Answer from the drawing. Dimensions are ordinates in mm from the lowest x, y and z of the part. Give positions to 0.01 mm unless a question says otherwise; leave off trailing zeros. Loops run counter-clockwise (first coordinate to the right, second up) from the corner with the lowest first, then second, coordinate; pieces in that order, holes last.
Item 1: The mould has two halves that part along Y. Classify the marked faces 1 and 2: pulls with the +Y half, pulls with the -Y half, needs draft (parallel to the pull), parting line crosses it, or undercut.
Item 2: Section A-A, the plane y = 15 is taken. Give the vertices of the cut face in (x, z), and give its area (3 significant figures).
Item 3: Section C-C, the plane z = 2.85 is taken. Give the vertices of the cut face in (x, y), and give its area (3 significant figures).
Item 4: Section D-D, the plane y = 69 is taken. Give the vertices of the cut face in (x, z), and give its area (3 significant figures).
Item 5: Section B-B, the plane x = 15 is taken. Give the vertices of the cut face in (y, z), and give its area (3 significant figures).
Item 6: Consider line 1 along Y through (x, z) = (15, 2.7); line 2 along Y through (x, z) = (10, 4.65); line 3 along X through (y, z) = (72.5, 3.7). Determine where each line is inside the solid, lowest interval first.
Item 7: Each of these flat-tipped pins is pushed along its axis until it touches: pin 1 Ø12 at (x, y) = (15, 15) entering from +Z; pin 2 Ø1 at (y, z) = (52, 3) entering from -X; pin 3 Ø3 at (y, z) = (68, 3) entering from +X. Where does it stop, or does it pass through?
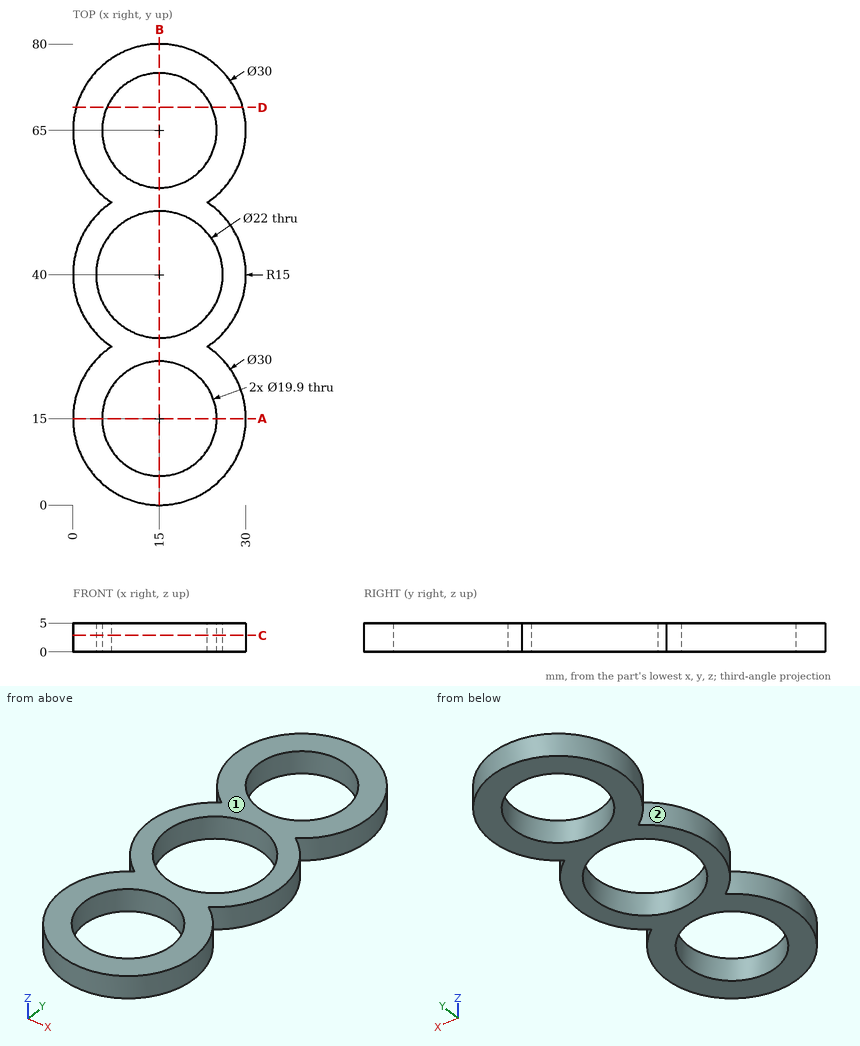
Worked answers:
1. face 1: needs draft
1. face 2: undercut
2. outline: (0, 0) - (5.05, 0) - (5.05, 5) - (0, 5) - close; (24.95, 0) - (30, 0) - (30, 5) - (24.95, 5) - close
2. area: 50.5 mm2
3. outline: (6.71, 27.5) arc R15 ccw (long way) to (23.29, 27.5) arc R15 ccw to (23.29, 52.5) arc R15 ccw (long way) to (6.71, 52.5) arc R15 ccw to start; hole circle Ø22 at (15, 40); hole circle Ø19.9 at (15, 15); hole circle Ø19.9 at (15, 65)
3. area: 1,010 mm2
4. outline: (0.54, 0) - (5.89, 0) - (5.89, 5) - (0.54, 5) - close; (24.11, 0) - (29.46, 0) - (29.46, 5) - (24.11, 5) - close
4. area: 53.5 mm2
5. outline: (0, 0) - (5.05, 0) - (5.05, 5) - (0, 5) - close; (24.95, 0) - (29, 0) - (29, 5) - (24.95, 5) - close; (51, 0) - (55.05, 0) - (55.05, 5) - (51, 5) - close; (74.95, 0) - (80, 0) - (80, 5) - (74.95, 5) - close
5. area: 91.0 mm2
6. line 1: y = 0 to 5.05, 24.95 to 29, 51 to 55.05, 74.95 to 80
6. line 2: y = 0.86 to 6.4, 23.6 to 30.2, 49.8 to 56.4, 73.6 to 79.14
6. line 3: x = 2.01 to 8.46, 21.54 to 27.99
7. pin 1: passes through
7. pin 2: stops at x = 5.37
7. pin 3: stops at x = 29.92
